The model under review builds one solid part; all positions refer to its coordinate system, in mm. A direction names the side the tool comes from. Give positions to 0.01 mm unless a question says otherwise; leave off trailing zeros. Order: outer loops, then holes, each group sorted by start corner. A loop starts at its lowest first (then second) coordinate and runs counter-clockwise, first axis right, second up. Notation, with made-up numbers: (27, 57.25) - (76, 57.25) arc R24 ccw to (76, 92.25) - close; hole circle Ø9 at (83.25, -2.75). An arc over 180 degrees is marked (long way). Use CSV: the item, a comma, the result in double quotes. Start each with the question number.
1. Take a section at B-B, the plane z = 16. State the section outline as (x, y) points, then the cut area to 3 significant figures.
2. For pin 1 (4 mm diameter, centred on y = -5, z = 12.5, fed in from -X); pin 2 (3 mm diameter, centred on x = 3, z = 10.5, fed in from -Y); pin 3 (8 mm diameter, centred on x = 6, z = 8, fed in from -Y), all flat-tipped, find the tip position at first contact; note any pin that passes through.
3. Draft analysis for pull direction X (two halves, no side actions). For faces 6 (the flat face through (5.324, 9.051, 23.944)), 7 (the flat face through (1, 7, 0)), 8 (the flat face through (-8, 3, 19.5)), state which applies: released by +X, released by -X, zero draft, split by the parting line, or undercut.
4. To check wall thickness, follow line 1 (Y direction, x = 0, z = 16.35); line 2 (X direction, y = 0, z = 20.15); line 3 (X direction, y = -2, z = 23.75). State the ranges of each line that lie inside material, in increasing order. Write a range as [from, to].
5. Machinability: for faces 1 (the flat face through (-8, -3, 28)), 2 (the flat face through (6, -2, 16.7)), 3 (the flat face through (-10.5, 0, 24)), 4 (the cylindrical face through (-8.584, -2.703, 18.021)), 5 (the cylindrical face through (-2.17, -9.76, 17.46)), which of the approach directions +Z, -Z, +X, -X, +Y, -Y give a long, thin tool a straight path to every point of the face, cutting with its end or side? Answer none if there is none.
6. Take a section at C-C, the plane z = 13. State the section outline as (x, y) points, then the cut area to 3 significant figures.
7. Take a section at A-A, the plane z = 4.5. Count the separate pieces of the cut face and the enclosed holes in it, then the cut area to 3 significant figures.
```python
from build123d import *

# Parameters (mm, degrees)
SKETCH_2_R               = 8.5
EXTRUDE_1_DEPTH          = 15
SKETCH_3_R               = 10
EXTRUDE_2_DEPTH          = 5
EXTRUDE_3_DEPTH          = 8
SKETCH_6_R               = 6.75
CUT_EXTRUDE_1_DEPTH      = 15
SKETCH_7_R               = 5.9
CUT_EXTRUDE_2_DEPTH      = 22.960191256
M18X1_5_1_D              = 16.5
M18X1_5_1_DEPTH          = 7
M18X1_5_1_TIP            = 4.957100107
CUT_EXTRUDE_START        = 19.5
SKETCH_13_R              = 8.25
CUT_EXTRUDE_3_DEPTH      = 1.5
SWEEP_1_PROFILE_R        = 0.6
PATTERN_CIRCULAR_1_COUNT = 5


with BuildPart() as part:
    # 草图2 → 凸台-拉伸1 (new body)
    with BuildSketch(Plane.XY):
        Circle(SKETCH_2_R)
    extrude(amount=EXTRUDE_1_DEPTH)

    # 草图3 → 凸台-拉伸2 (add)
    with BuildSketch(Plane.XY.offset(15)):
        Circle(SKETCH_3_R)
    extrude(amount=EXTRUDE_2_DEPTH)

    # 草图4 → 凸台-拉伸3 (add)
    with BuildSketch(Plane.XY.offset(20)):
        Polygon((0, 12.124355653), (-10.5, 6.062177826), (-10.5, -6.062177826), (0, -12.124355653), (10.5, -6.062177826), (10.5, 6.062177826), align=None)
    extrude(amount=EXTRUDE_3_DEPTH)

    # 草图6 → 切除-拉伸1 (cut)
    with BuildSketch(Plane(origin=(0, 0, 0), x_dir=(-1, 0, 0), z_dir=(0, 0, -1))):
        Circle(SKETCH_6_R)
    extrude(amount=-CUT_EXTRUDE_1_DEPTH, mode=Mode.SUBTRACT)

    # 草图7 → 切除-拉伸2 (cut, through all)
    with BuildSketch(Plane(origin=(0, 0, 15), x_dir=(-1, 0, 0), z_dir=(0, 0, -1))):
        Circle(SKETCH_7_R)
    extrude(amount=-CUT_EXTRUDE_2_DEPTH, mode=Mode.SUBTRACT)

    # 草图8 → 切除-旋转1 (revolve, cut)
    with BuildSketch(Plane(origin=(0, 0, 0), x_dir=(0, 0, -1), z_dir=(1, 0, 0)), mode=Mode.PRIVATE) as cut_revolve_1_sk:
        Polygon((-16.7, 0), (-16.7, -6.9), (-16.5, -6.9), (-16.5, -9), (-19.5, -9), (-19.5, 0), align=None)
    revolve(cut_revolve_1_sk.sketch.rotate(Axis((0, 0, 5.279548329), (0, 0, 1)), 270), axis=Axis((0, 0, 5.279548329), (0, 0, 1)), mode=Mode.SUBTRACT)

    # M18x1.5 螺纹孔1
    with Locations(Plane.XY.offset(28)):
        with Locations((0, 0)):
            Hole(M18X1_5_1_D / 2, depth=M18X1_5_1_DEPTH)
            with Locations((0, 0, -(M18X1_5_1_DEPTH + M18X1_5_1_TIP / 2))):  # 118° drill point
                Cone(0, M18X1_5_1_D / 2, M18X1_5_1_TIP, mode=Mode.SUBTRACT)

    # 草图13 → 切除-拉伸3 (cut)
    with BuildSketch(Plane.XY.offset(CUT_EXTRUDE_START)):
        Circle(SKETCH_13_R)
    extrude(amount=CUT_EXTRUDE_3_DEPTH, mode=Mode.SUBTRACT)

    # 切除-扫描1: sweep along a path in 草图14
    with BuildLine(Plane.XY.offset(2)) as sweep_1_path:
        CenterArc((0, 0), 8.5, 0, 360)
    # 切除-扫描1 profile (on start of the path) → 切除-扫描1 (sweep, cut)
    with BuildSketch(Plane(origin=(8.5, 0, 2), x_dir=(0, 0, 1), z_dir=(0, 1, 0))):
        Circle(SWEEP_1_PROFILE_R)
    sweep(path=sweep_1_path.line, mode=Mode.SUBTRACT)

    # 草图22 → Ø3.1 (3.1) 直径孔1 (revolve, cut)
    with BuildSketch(Plane(origin=(0, 8.5, 4.5), x_dir=(0, 0, 1), z_dir=(1, 0, 0))):
        Polygon((0, 0), (0, 4.184678752), (1.55, 1.5), (1.55, 0), align=None)
    hole_wizard_3_1_3_1_1 = revolve(axis=Axis((0, 14.85, 4.5), (0, -1, 0)), mode=Mode.SUBTRACT)

    # 阵列(圆周)1: Ø3.1 (3.1) 直径孔1 ×5 about axis
    pattern_circular_1_axis = Axis((0, 0, 0), (0, 0, 1))
    for i in range(1, PATTERN_CIRCULAR_1_COUNT):
        add(hole_wizard_3_1_3_1_1.rotate(pattern_circular_1_axis, i * 360 / PATTERN_CIRCULAR_1_COUNT), mode=Mode.SUBTRACT)


solid = part.part
```
Determined:
1,outline,"circle Ø20 at (0, 0); hole circle Ø11.8 at (0, 0)"
1,area,"205 mm²"
2,pin 1,"stops at x = -7.95"
2,pin 2,"stops at y = -8.37"
2,pin 3,"stops at y = -8.26"
3,face 6,"released by +X"
3,face 7,"zero draft"
3,face 8,"undercut"
4,line 1,"y = [-10, -5.9], [5.9, 10]"
4,line 2,"x = [-10.5, -8.25], [8.25, 10.5]"
4,line 3,"x = [-10.5, -8], [8, 10.5]"
5,face 1,"+Z, +X, -X, +Y, -Y"
5,face 2,"+Z"
5,face 3,"+Z, -Z, -X, +Y, -Y"
5,face 4,"none"
5,face 5,"-Z"
6,outline,"circle Ø17 at (0, 0); hole circle Ø13.5 at (0, 0)"
6,area,"83.8 mm²"
7,separate pieces,"5"
7,enclosed holes,"0"
7,area,"57.0 mm²"
